```python
from build123d import *

# Parameters (mm, degrees)
ESQUISSE1_R                    = 55
ESQUISSE1_R_2                  = 45.25
BOSS_EXTRU_1_DEPTH             = 5
BOSS_EXTRU_2_DEPTH             = 5
BOSS_EXTRU_3_REACH             = 118.795
BOSS_EXTRU_3_DIRECTION_2_REACH = 118.795
CONG_1_R                       = 5
CONG_2_R                       = 5
CONG_3_R                       = 5
BOSS_EXTRU_4_DEPTH             = 7
BOSS_EXTRU_5_DEPTH             = 5
CONG_7_R                       = 20


with BuildPart() as part:
    # Esquisse1 → Boss.-Extru.1 (new body)
    with BuildSketch(Plane.XY):
        Circle(ESQUISSE1_R)
        Circle(ESQUISSE1_R_2, mode=Mode.SUBTRACT)
    extrude(amount=BOSS_EXTRU_1_DEPTH)

    # Esquisse2 → Boss.-Extru.2 (add)
    with BuildSketch(Plane(origin=(0, 0, 0), x_dir=(-1, 0, 0), z_dir=(0, 0, -1))):
        with BuildLine():
            Line((-50, -22.912878475), (-50, -102.912878475))
            Line((-50, -102.912878475), (50, -102.912878475))
            Line((50, -102.912878475), (50, -22.912878475))
            ThreePointArc((50, -22.912878475), (0, -55), (-50, -22.912878475))
        make_face()
    extrude(amount=-BOSS_EXTRU_2_DEPTH)

    # Boss.-Extru.3: up to this face of the body (flat: up to its plane)
    boss_extru_3_end = Plane(part.part.faces().sort_by_distance((50, -62.912878475, 2.5))[0])
    # Esquisse3 → Boss.-Extru.3 (add, up to the picked face)
    with BuildSketch(Plane(origin=(0, 0, 0), x_dir=(0, 0, -1), z_dir=(1, 0, 0)), mode=Mode.PRIVATE) as boss_extru_3_sk1:
        with BuildLine():
            Line((-5, -102.912878475), (-57.400351245, -67.211308793))
            Line((-57.400351245, -67.211308793), (-54.585063802, -63.079220143))
            ThreePointArc((-54.585063802, -63.079220143), (-54.440259998, -62.937915144), (-54.251927212, -62.863982707))
            Line((-54.251927212, -62.863982707), (-5, -54.179539087))
            Line((-5, -54.179539087), (-5, -59.256672147))
            Line((-5, -59.256672147), (-35.834324462, -64.693595481))
            ThreePointArc((-35.834324462, -64.693595481), (-38.617179929, -67.272281909), (-37.416008291, -70.871044883))
            Line((-37.416008291, -70.871044883), (-5, -96.86266946))
            Line((-5, -96.86266946), (-5, -102.912878475))
        make_face()
    boss_extru_3_tool1 = split(extrude(boss_extru_3_sk1.sketch, amount=BOSS_EXTRU_3_REACH, mode=Mode.PRIVATE), bisect_by=boss_extru_3_end, keep=Keep.BOTH, mode=Mode.PRIVATE)
    add(boss_extru_3_tool1.solids().sort_by(Axis((0, -84.470715, 30.797256), (1, 0, 0)))[0])

    # Boss.-Extru.3 direction 2: up to this face of the body (flat: up to its plane)
    boss_extru_3_direction_2_end = Plane(part.part.faces().sort_by_distance((-50, -62.912878475, 2.5))[0])
    # Esquisse3 → Boss.-Extru.3 direction 2 (add, up to the picked face)
    with BuildSketch(Plane(origin=(0, 0, 0), x_dir=(0, 0, -1), z_dir=(1, 0, 0)), mode=Mode.PRIVATE) as boss_extru_3_direction_2_sk1:
        with BuildLine():
            Line((-5, -102.912878475), (-57.400351245, -67.211308793))
            Line((-57.400351245, -67.211308793), (-54.585063802, -63.079220143))
            ThreePointArc((-54.585063802, -63.079220143), (-54.440259998, -62.937915144), (-54.251927212, -62.863982707))
            Line((-54.251927212, -62.863982707), (-5, -54.179539087))
            Line((-5, -54.179539087), (-5, -59.256672147))
            Line((-5, -59.256672147), (-35.834324462, -64.693595481))
            ThreePointArc((-35.834324462, -64.693595481), (-38.617179929, -67.272281909), (-37.416008291, -70.871044883))
            Line((-37.416008291, -70.871044883), (-5, -96.86266946))
            Line((-5, -96.86266946), (-5, -102.912878475))
        make_face()
    boss_extru_3_direction_2_tool1 = split(extrude(boss_extru_3_direction_2_sk1.sketch, amount=-BOSS_EXTRU_3_DIRECTION_2_REACH, mode=Mode.PRIVATE), bisect_by=boss_extru_3_direction_2_end, keep=Keep.BOTH, mode=Mode.PRIVATE)
    add(boss_extru_3_direction_2_tool1.solids().sort_by(Axis((0, -84.470715, 30.797256), (-1, 0, 0)))[0])

    # Congé1
    cong_1_edges = [part.edges().sort_by_distance(p)[0] for p in [
        (0, -59.256672147, 5),
    ]]
    fillet(cong_1_edges, radius=CONG_1_R)

    # Congé2
    cong_2_edges = [part.edges().sort_by_distance(p)[0] for p in [
        (0, -54.179539087, 5),
    ]]
    fillet(cong_2_edges, radius=CONG_2_R)

    # Congé3
    cong_3_edges = [part.edges().sort_by_distance(p)[0] for p in [
        (0, -96.86266946, 5),
    ]]
    fillet(cong_3_edges, radius=CONG_3_R)

    # Esquisse5 → Boss.-Extru.4 (add)
    with BuildSketch(Plane(origin=(50, 0, 0), x_dir=(0, 0, -1), z_dir=(1, 0, 0))):
        with BuildLine():
            Line((-9.131759112, -54.908079696), (-54.251927212, -62.863982707))
            ThreePointArc((-54.251927212, -62.863982707), (-54.440259998, -62.937915144), (-54.585063802, -63.079220143))
            Line((-54.585063802, -63.079220143), (-57.400351245, -67.211308793))
            Line((-57.400351245, -67.211308793), (-5, -102.912878475))
            Line((-5, -102.912878475), (0, -102.912878475))
            Line((0, -102.912878475), (0, -22.912878475))
            Line((0, -22.912878475), (-5, -22.912878475))
            Line((-5, -22.912878475), (-5, -49.984040931))
            ThreePointArc((-5, -49.984040931), (-6.169777784, -53.19797898), (-9.131759112, -54.908079696))
        make_face()
        with BuildLine():
            Line((-35.834324462, -64.693595481), (-10.868240888, -60.291401345))
            ThreePointArc((-10.868240888, -60.291401345), (-6.786061952, -61.385217894), (-5, -65.21544011))
            Line((-5, -65.21544011), (-5, -86.444801488))
            ThreePointArc((-5, -86.444801488), (-7.836547445, -90.952514105), (-13.127789216, -90.34569044))
            Line((-13.127789216, -90.34569044), (-37.416008291, -70.871044883))
            ThreePointArc((-37.416008291, -70.871044883), (-38.617179929, -67.272281909), (-35.834324462, -64.693595481))
        make_face(mode=Mode.SUBTRACT)
    extrude(amount=BOSS_EXTRU_4_DEPTH)

    # Esquisse6 → Boss.-Extru.5 (add, through all)
    with BuildSketch(Plane.XY.offset(5)):
        with BuildLine():
            Line((57, -22.912878475), (52.753659593, -15.558001143))
            ThreePointArc((52.753659593, -15.558001143), (51.508273074, -19.284652056), (50, -22.912878475))
            Line((50, -22.912878475), (57, -22.912878475))
        make_face()
    extrude(amount=-BOSS_EXTRU_5_DEPTH)

    # Congé7
    cong_7_edges = [part.edges().sort_by_distance(p)[0] for p in [
        (57, -22.912878475, 2.5),
    ]]
    fillet(cong_7_edges, radius=CONG_7_R)


solid = part.part
```
Geometry check sheet. Reference: the model listing, model coordinates, mm. A direction names the side the tool comes from. Give positions to 0.01 mm unless a question says otherwise; leave off trailing zeros. Order: outer loops, then holes, each group sorted by start corner. A loop starts at its lowest first (then second) coordinate and runs counter-clockwise, first axis right, second up.
1. Thickness scan on L1, parallel to Y at x = 0, z = 2.9; L2, parallel to Y at x = 31, z = 4; L3, parallel to Z at x = -21, y = -46. Record the ranges inside material, lowest first.
2. Section check C-C, the plane z = 29. Enter the section's corners in (x, y), and give its area (3 significant figures).
3. Section check A-A, the plane x = 0. Enter the section's corners in (y, z), and give its area (3 significant figures).
4. Section check D-D, the plane x = -29.5. Enter the section's corners in (y, z), and give its area (3 significant figures).
5. Access from +Z, -Z, +X, -X, +Y, -Y to the whole of each face (thin tool, end or side, straight path). Record for faces 4 (the face through (-50, -60, 22)), 5 (the face through (2.75, -67.33, 38.63)), 6 (the face through (21.5, -40, 5)).
6. Section check B-B, the plane y = 0. Enter the section's corners in (x, z), and give its area (3 significant figures).
7. Release check for a two-part mould opening along Y. For faces 1 (the face through (2.751, -65.116, 55.973)), 2 (the face through (57, -62.7, 26.7)), 3 (the face through (43.16, 13.59, 2.46)) record: pulls with the +Y half, pulls with the -Y half, needs draft (parallel to the pull), parting line crosses it, or undercut.
8. Gauge pin test, flat ends, axial feed: pin 1 Ø8 at (x, z) = (-38, 49.5) entering from +Y; pin 2 Ø4 at (x, z) = (37, 23.5) entering from +Y; pin 3 Ø1.5 at (x, z) = (19, 16) entering from +Y. Record the tip position at first contact, or that the pin passes through.
Values follow:
1. L1: y = -102.91 to -45.25, 45.25 to 55
1. L2: y = -102.91 to -32.96, 32.96 to 45.43
1. L3: z = 0 to 5
2. outline: (-50, -86.56) - (57, -86.56) - (57, -77.62) - (-50, -77.62) - close; (-50, -63.49) - (57, -63.49) - (57, -58.41) - (-50, -58.41) - close
2. area: 1,500 mm2
3. outline: (-102.91, 0) - (-45.25, 0) - (-45.25, 5) - (-49.98, 5) arc R5 cw to (-54.91, 9.13) - (-62.86, 54.25) arc R0.51 ccw to (-63.08, 54.59) - (-67.21, 57.4) - (-102.91, 5) - close; (45.25, 0) - (55, 0) - (55, 5) - (45.25, 5) - close; hole (-90.35, 13.13) arc R5 ccw to (-86.44, 5) - (-65.22, 5) arc R5 ccw to (-60.29, 10.87) - (-64.69, 35.83) arc R3.5 ccw to (-70.87, 37.42) - close
3. area: 1,030 mm2
4. outline: (-102.91, 0) - (-34.31, 0) - (-34.31, 5) - (-49.98, 5) arc R5 cw to (-54.91, 9.13) - (-62.86, 54.25) arc R0.51 ccw to (-63.08, 54.59) - (-67.21, 57.4) - (-102.91, 5) - close; (34.31, 0) - (46.42, 0) - (46.42, 5) - (34.31, 5) - close; hole (-90.35, 13.13) arc R5 ccw to (-86.44, 5) - (-65.22, 5) arc R5 ccw to (-60.29, 10.87) - (-64.69, 35.83) arc R3.5 ccw to (-70.87, 37.42) - close
4. area: 1,100 mm2
5. face 4: +Z, -Z, -X, -Y
5. face 5: +X, -X
5. face 6: +Z, +X, -X, +Y
6. outline: (-55, 0) - (-45.25, 0) - (-45.25, 5) - (-55, 5) - close; (45.25, 0) - (55, 0) - (55, 5) - (45.25, 5) - close
6. area: 97.5 mm2
7. face 1: pulls with the +Y half
7. face 2: needs draft
7. face 3: undercut
8. pin 1: stops at y = -61.32
8. pin 2: stops at y = -57.09
8. pin 3: stops at y = -55.99
